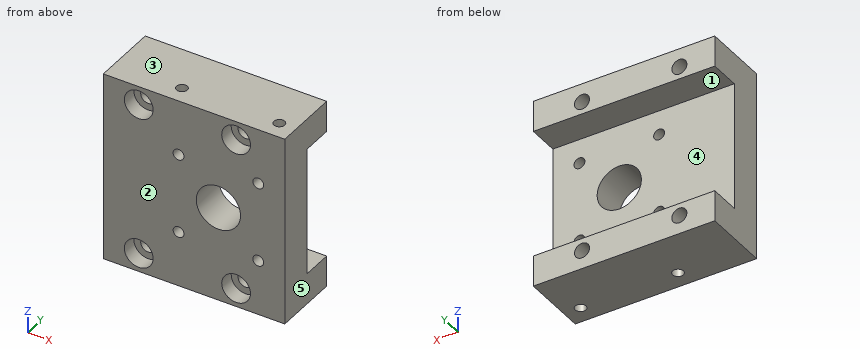
Autodesk Inventor part; units mm, degrees
ref_plane "Arbeitsebene1" through (-34, 0, 0) normal (0, 0, 1) x (1, 0, 0)
ref_plane "Arbeitsebene2" through (27, 0, 0) normal (0, 0, -1) x (-1, 0, 0)
ref_plane "YZ Plane" through (0, 0, 0) normal (1, 0, 0) x (0, 1, 0)
sketch "Skizze1" plane through (0, 0, 0) normal (0, 1, 0) x (-1, 0, 0)
  line L0 (-34, 21.5) -> (34, 21.5)
  line L1 (34, 21.5) -> (34, -21.5)
  line L2 (34, -21.5) -> (-34, -21.5)
  line L3 (-34, -21.5) -> (-34, 21.5)
  line L4 (-34, 21.5) -> (34, -21.5) construction
  line L5 (34, 21.5) -> (-34, -21.5) construction
  point P0 (0, 0)
  dimension "d0" = 43
  dimension "d1" = 68
extrude "Extrusion1" add sketch "Skizze1" along normal blind 15
sketch "Skizze2" plane through (0, 15, 0) normal (0, 1, 0) x (1, 0, 0)
  line L0 (-34, -21.5) -> (34, -21.5)
  line L1 (34, -21.5) -> (34, 21.5)
  line L2 (34, 21.5) -> (-34, 21.5)
  line L3 (-34, 21.5) -> (-34, -21.5)
  line L4 (-34, 14.5) -> (27, 14.5)
  line L5 (27, 14.5) -> (27, -14.5)
  line L6 (27, -14.5) -> (-34, -14.5)
  line L7 (-34, -14.5) -> (-34, 14.5)
  point P0 (0, 0)
  dimension "d4" = 29
  dimension "d5" = 14.5
  dimension "d9" = 7
  dimension "d10" = 7
extrude "Extrusion2" cut sketch "Skizze2" against normal blind 7 contours L3 L4 L5 L6
sketch "Skizze3" plane through (0, 0, 0) normal (0, -1, 0) x (1, 0, 0)
  line L0 (-34, 14.5) -> (-34, -14.5)
  line L1 (27, 14.5) -> (-34, 14.5)
  line L2 (27, -14.5) -> (27, 14.5)
  line L3 (-34, -14.5) -> (27, -14.5)
  circle A0 centre (12, 0) radius 5
  line L4 (0, 0) -> (50.6239, 0) construction
  point P0 (16, 17.3)
  dimension "d11" = 11
  dimension "d12" = 17.3
  dimension "d24" = 10
  dimension "d27" = 4
hole "Bohrung1" at (16, 0, 17.3) direction (0, 1, 0) diameter 3.4 end through all counterbore diameter 6.5 counterbore depth 3.4
pattern_linear "Rechteckige Anordnung1" count 3 spacing 22 along (-1, 0, 0) of "Bohrung1"
ref_plane "Arbeitsebene1" through (-34, 0, 0) normal (0, 0, 1) x (1, 0, 0)
mirror "Spiegeln1" about plane through (-34, 0, 0) normal (0, 0, 1) of "Bohrung1", "Rechteckige Anordnung1"
extrude "Extrusion3" cut sketch "Skizze3" against normal through all contours A0
sketch "Skizze4" plane through (0, 8, 0) normal (0, 1, 0) x (1, 0, 0)
  circle A0 centre (12, 0) radius 5
  line L0 (-34, -14.5) -> (-34, 14.5)
  line L1 (27, -14.5) -> (-34, -14.5)
  line L2 (27, 14.5) -> (27, -14.5)
  line L3 (-34, 14.5) -> (27, 14.5)
  line L4 (21, -9) -> (3, -9)
  line L5 (3, -9) -> (3, 9)
  line L6 (3, 9) -> (21, 9)
  line L7 (21, 9) -> (21, -9)
  line L8 (21, -9) -> (3, 9) construction
  line L9 (3, -9) -> (21, 9) construction
  point P0 (0, 0)
  dimension "d28" = 18
  dimension "d29" = 18
hole "Bohrung2" at (3, 8, 9) at (3, 8, -9) at (21, 8, -9) at (21, 8, 9) direction (0, -1, 0) diameter 2.459 depth 8.8 tip angle 118
sketch "Skizze5" plane through (0, 15, 0) normal (0, 1, 0) x (1, 0, 0)
  circle A0 centre (-28, 17.3) radius 1.7
  circle A1 centre (-6, 17.3) radius 1.7
  circle A2 centre (16, 17.3) radius 1.7
  circle A3 centre (-28, -17.3) radius 1.7
  circle A4 centre (-6, -17.3) radius 1.7
  circle A5 centre (16, -17.3) radius 1.7
  line L0 (27, -14.5) -> (-34, -14.5)
  line L1 (-34, -14.5) -> (-34, -21.5)
  line L2 (-34, -21.5) -> (34, -21.5)
  line L3 (34, -21.5) -> (34, 21.5)
  line L4 (34, 21.5) -> (-34, 21.5)
  line L5 (-34, 21.5) -> (-34, 14.5)
  line L6 (-34, 14.5) -> (27, 14.5)
  line L7 (27, 14.5) -> (27, -14.5)
  line L8 (-34, 21.5) -> (34, 21.5)
  line L9 (34, -21.5) -> (27, -21.5)
  line L10 (27, -21.5) -> (27, 21.5)
  line L11 (27, 21.5) -> (34, 21.5)
  line L12 (34, 21.5) -> (34, -21.5)
  point P0 (0, 0)
extrude "Extrusion4" cut sketch "Skizze5" against normal through all contours L7 L10 L4 L3 L2
sketch "Skizze6" plane through (-34, 0, -21.5) normal (-1, 0, 0) x (0, 0, 1)
  line L0 (36, 15) -> (36, 8)
  line L1 (36, 8) -> (7, 8)
  line L2 (7, 8) -> (7, 15)
  line L3 (0, 15) -> (7, 15)
  line L4 (0, 0) -> (0, 15)
  line L5 (43, 0) -> (0, 0)
  line L6 (43, 0) -> (43, 15)
  line L7 (36, 15) -> (43, 15)
  point P0 (21.5, 0)
extrude "Extrusion5" cut sketch "Skizze6" against normal blind 20
sketch "Skizze7" plane through (27, 0, -21.5) normal (0, 0, -1) x (-1, 0, 0)
  line L0 (34.7, 3.4) -> (31.3, 3.4)
  line L1 (36.25, 3.4) -> (29.75, 3.4)
  line L2 (31.3, 15) -> (34.7, 15)
  line L3 (9.3, 15) -> (12.7, 15)
  line L4 (14.25, 3.4) -> (7.75, 3.4)
  line L5 (34.7, 15) -> (34.7, 3.4)
  line L6 (34.7, 3.4) -> (34.7, 15)
  line L7 (31.3, 15) -> (31.3, 3.4)
  line L8 (9.3, 3.4) -> (12.7, 3.4)
  line L9 (12.7, 15) -> (12.7, 3.4)
  line L10 (9.3, 15) -> (9.3, 3.4)
  line L11 (0, 8) -> (41, 8)
  line L12 (29.75, 3.4) -> (29.75, 0)
  line L13 (29.75, 0) -> (29.75, 3.4)
  line L14 (29.75, 3.4) -> (36.25, 3.4)
  line L15 (36.25, 3.4) -> (36.25, 0)
  line L16 (36.25, 0) -> (36.25, 3.4)
  line L17 (14.25, 3.4) -> (14.25, 0)
  line L18 (14.25, 3.4) -> (14.25, 0)
  line L19 (7.75, 3.4) -> (14.25, 3.4)
  line L20 (7.75, 3.4) -> (7.75, 0)
  line L21 (7.75, 3.4) -> (7.75, 0)
  line L22 (41, 0) -> (0, 0)
  point P0 (27, 0)
  point P1 (25.75, 4)
  point P2 (3.75, 4)
  dimension "d41" = 8
  dimension "d42" = 4
  dimension "d43" = 4
  dimension "d44" = 4
  dimension "d45" = 4
hole "Bohrung3" at (1.25, 4, -21.5) at (23.25, 4, -21.5) direction (0, 0, 1) diameter 2.459 depth 8.8 tip angle 118
ref_plane "Arbeitsebene2" through (27, 0, 0) normal (0, 0, -1) x (-1, 0, 0)
mirror "Spiegeln2" about plane through (27, 0, 0) normal (0, 0, -1) of "Bohrung3"
equation "\"d10\" = d9"
equation "\"d29\" = d28"
properties part number "connection_hand_2" material "Aluminium 6061"
The listing builds one solid part. Answer for the finished solid, in the listing's coordinates (mm). Face numbers are marked on the shaded views. A direction names the side the tool comes from. Round coordinates to 2 decimals unless told otherwise and drop trailing zeros. Write each loop counter-clockwise with the first axis right and the second up, starting at its lowest first coordinate (ties: lowest second). Pieces come first, ordered by that corner, then holes. Notation, with made-up numbers: M 84.25,75 L 104.25,75 A32 ccw 104.25,110 Z; hole C -5.75,15 d8. An arc over 180 degrees is marked long. Write each question's results on one line, items separated by ' | '. Start each with the question number.
Item 1: Straight lines are drawn through the part: probe 1 along Z at (x, y) = (-6, 9.5); probe 2 along X at (y, z) = (3.5, 9); probe 3 along Z at (x, y) = (21, 6.5). For each, find the intervals that lie inside material, in ascending order.
Item 2: Find section B-B on x = -6. Write down the section's boundary in (y, z).
Item 3: The mould has two halves that part along Z. Classify the marked faces 3, 4 and 5: +Z half, -Z half, draft (parallel to the pull), parting line (faces both ways), or undercut.
Item 4: Given pin 1 Ø2 at (x, z) = (21, 9) entering from +Y; pin 2 Ø1 at (x, z) = (0, -4) entering from +Y; pin 3 Ø6 at (x, z) = (-6, -17.3) entering from -Y; pin 4 Ø2 at (x, y) = (1.25, 4) entering from +Z, each flat-ended and moving along its own axis, determine where each tip first touches the part or whether it passes through.
Item 5: Find section A-A on z = -17.3. Write down the section's boundary in (x, y).
Item 6: Find section D-D on z = -3. Write down the section's boundary in (x, y).
Item 7: Which of the six approach directions +Z, -Z, +X, -X, +Y, -Y give full straight-line access (tool end or side, diameter ignored) to the marked faces 1 and 2?
Item 8: Find section C-C on y = 13.25. Write down the section's boundary in (x, z), and give its area (3 significant figures).
Answer block:
1) probe 1: z = -21.5 to -19, -15.6 to -14.5, 14.5 to 15.6, 19 to 21.5 | probe 2: x = -14 to 1.77, 4.23 to 19.77, 22.23 to 27 | probe 3: z = -21.5 to -10.23, -7.77 to 7.77, 10.23 to 21.5
2) outline: M 0,-21.5 L 15,-21.5 L 15,-19 L 3.4,-19 L 3.4,-20.55 L 0,-20.55 Z; M 0,-14.05 L 3.4,-14.05 L 3.4,-15.6 L 15,-15.6 L 15,-14.5 L 8,-14.5 L 8,14.5 L 15,14.5 L 15,15.6 L 3.4,15.6 L 3.4,14.05 L 0,14.05 Z; M 0,20.55 L 3.4,20.55 L 3.4,19 L 15,19 L 15,21.5 L 0,21.5 Z
3) face 3: +Z half | face 4: undercut | face 5: draft
4) pin 1: passes through | pin 2: stops at y = 8 | pin 3: stops at y = 3.4 | pin 4: stops at z = 12.56
5) outline: M -14,0 L -9.25,0 L -9.25,3.4 L -7.7,3.4 L -7.7,15 L -14,15 Z; M -4.3,3.4 L -2.75,3.4 L -2.75,0 L 12.75,0 L 12.75,3.4 L 14.3,3.4 L 14.3,15 L -4.3,15 Z; M 17.7,3.4 L 19.25,3.4 L 19.25,0 L 27,0 L 27,15 L 17.7,15 Z; hole C 1.25,4 d2.46; hole C 23.25,4 d2.46
6) outline: M -14,0 L 8,0 L 8,8 L -14,8 Z; M 16,0 L 27,0 L 27,8 L 16,8 Z
7) face 1: +X, -X, +Y | face 2: +Z, -Z, +X, -X, -Y
8) outline: M -14,-21.5 L 27,-21.5 L 27,-14.5 L -14,-14.5 Z; M -14,14.5 L 27,14.5 L 27,21.5 L -14,21.5 Z; hole C -6,-17.3 d3.4; hole C -6,17.3 d3.4; hole C 16,-17.3 d3.4; hole C 16,17.3 d3.4 | area: 538 mm²
